The model under review builds one solid part; all positions refer to its coordinate system, in mm. A direction names the side the tool comes from. Coordinates: 2 decimals unless noted, no trailing zeros. Write each loop counter-clockwise with the first axis right and the second up, starting at its lowest first coordinate (ties: lowest second). Pieces come first, ordered by that corner, then holes. Notation, with made-up numbers: (23.5, 75) - (29.5, 75) arc R30 ccw to (29.5, 112) - close; hole circle Ø1 at (56.25, 57). An arc over 180 degrees is marked (long way). Put each result on its own line as item: value.
Autodesk Inventor part; units mm, degrees
ref_plane "YZ Plane" through (0, 0, 0) normal (1, 0, 0) x (0, 1, 0)
ref_plane "XZ Plane" through (0, 0, 0) normal (0, 1, 0) x (-1, 0, 0)
ref_plane "XY Plane" through (0, 0, 0) normal (0, 0, 1) x (1, 0, 0)
sketch "Sketch2" plane through (0, 0, 0) normal (1, 0, 0) x (0, 1, 0)
  line L0 (26.4, -3) -> (6, -3)
  line L1 (6, -3) -> (6, -23.4)
  line L2 (6, -23.4) -> (26.4, -23.4)
  line L3 (26.4, -23.4) -> (26.4, -3)
  line L4 (30.4, 0) -> (0, 0)
  line L5 (30.4, -26.4) -> (30.4, 0)
  line L6 (0, 0) -> (0, -26.4)
  line L7 (30.4, -26.4) -> (0, -26.4)
  line L8 (6, -11) -> (0, -11)
  line L9 (0, -11) -> (0, -15.4)
  line L10 (0, -15.4) -> (6, -15.4)
  line L11 (6, -15.4) -> (6, -11)
  point P0 (0, -11)
  dimension "d5" = 20.4
  dimension "d6" = 20.4
  dimension "d8" = 6
  dimension "d22" = 4
  dimension "d23" = 3
  dimension "d24" = 3
  dimension "d27" = 8
  dimension "d28" = 8
extrude "Extrusion1" add sketch "Sketch2" along normal blind 54.8 contours L0 L1 L8 L6 L4 L5 L7 L10 L2 L3
sketch "Sketch13" plane through (0, 30.4, 0) normal (0, 1, 0) x (1, 0, 0)
  line L0 (0, 0) -> (54.8, 0)
  line L1 (0, 26.4) -> (54.8, 26.4)
  line L2 (54.8, 0) -> (50.8, 0)
  line L3 (50.8, 0) -> (50.8, 26.4)
  line L4 (50.8, 26.4) -> (54.8, 26.4)
  line L5 (54.8, 26.4) -> (54.8, 0)
  line L6 (4, 0) -> (0, 0)
  line L7 (0, 0) -> (0, 26.4)
  line L8 (0, 26.4) -> (4, 26.4)
  line L9 (4, 26.4) -> (4, 0)
  line L10 (0, 26.4) -> (0, 0)
  point P0 (0, 0)
  point P1 (69.8, 0)
  point P2 (69.8, 26.4)
  point P3 (4, 0)
  point P4 (54.8, 26.4)
  point P5 (50.8, 0)
  dimension "d75" = 4
  dimension "d76" = 4
  dimension "d77" = 46.8
extrude "Extrusion11" add sketch "Sketch13" along normal blind 27 contours L7 L1 L9 L0 | L3 L1 L5 L0
sketch "Sketch14" plane through (54.8, 30.4, 0) normal (1, 0, 0) x (0, 0, -1)
  circle A0 centre (5.2, 11) radius 1.3
  circle A1 centre (5.2, 23) radius 1.3
  line L0 (0, -30.4) -> (0, 27)
  circle A2 centre (21.2, 23) radius 1.3
  circle A3 centre (21.2, 11) radius 1.3
  line L1 (26.4, -30.4) -> (26.4, 27)
  line L2 (0, 0) -> (26.4, 0)
  point P0 (26.4, -4)
  dimension "d80" = 2.6
  dimension "d82" = 2.6
  dimension "d86" = 2.6
  dimension "d87" = 2.6
  dimension "d95" = 16
  dimension "d96" = 16
  dimension "d97" = 5.2
  dimension "d98" = 5.2
  dimension "d99" = 5.2
  dimension "d100" = 5.2
  dimension "d101" = 11
  dimension "d102" = 23
extrude "Extrusion12" cut sketch "Sketch14" against normal blind 100
ref_plane "Work Plane1" through (0, 0, -13.2) normal (0, 0, 1) x (1, 0, 0)
sketch "Sketch15" plane through (54.8, 0, 0) normal (1, 0, 0) x (0, 0, -1)
  line L0 (3, 26.4) -> (23.4, 26.4)
  line L1 (26.4, 30.4) -> (0, 30.4)
  line L2 (0, 30.4) -> (26.4, 30.4)
  line L3 (-2.8, 30.4) -> (29.2, 30.4)
  line L4 (29.2, 30.4) -> (29.2, 26.4)
  line L5 (29.2, 26.4) -> (-2.8, 26.4)
  line L6 (-2.8, 26.4) -> (-2.8, 30.4)
  line L7 (13.2, -11.48) -> (13.2, 68.88)
  line L8 (3, 26.4) -> (23.4, 26.4)
  point P0 (0, 0)
  point P1 (13.2, 30.4)
  point P2 (0, 30.4)
  dimension "d103" = 32
extrude "Extrusion13" add sketch "Sketch15" along normal blind 20 and the other way blind 75
sketch "Sketch16" plane through (-20.2, 30.4, 2.8) normal (0, 1, 0) x (1, 0, 0)
  line L0 (0, 32) -> (0, 0)
  line L1 (95, 0) -> (95, 32)
  line L2 (0, 0) -> (95, 0)
  line L3 (95, 0) -> (95, 2.8)
  line L4 (95, 2.8) -> (0, 2.8)
  line L5 (0, 2.8) -> (0, 0)
  line L6 (24.2, 29.2) -> (20.2, 29.2)
  line L7 (20.2, 29.2) -> (20.2, 2.8)
  line L8 (20.2, 2.8) -> (24.2, 2.8)
  line L9 (24.2, 2.8) -> (24.2, 29.2)
  line L10 (75, 29.2) -> (71, 29.2)
  line L11 (71, 29.2) -> (71, 2.8)
  line L12 (71, 2.8) -> (75, 2.8)
  line L13 (75, 2.8) -> (75, 29.2)
  line L14 (0, 0) -> (95, 0)
  line L15 (24.2, 2.8) -> (71, 2.8)
  line L16 (71, 2.8) -> (71, 0)
  line L17 (71, 0) -> (24.2, 0)
  line L18 (24.2, 0) -> (24.2, 2.8)
  point P0 (20.2, 2.8)
  point P1 (71, 2.8)
extrude "Extrusion14" add sketch "Sketch16" along normal blind 27 contours L4 L18 L2 L0 | L16 L4 L1 L2
fillet "Fillet5" radius 3 4 edges at (54.8, 30.4, -13.2) (64.8, 30.4, 0) (0, 30.4, -13.2) (-10.1, 30.4, 0)
sketch "Sketch17" plane through (54.8, 0, 0) normal (1, 0, 0) x (0, 0, -1)
  line L0 (-14.3714, 26.4) -> (47.2508, 26.4)
  line L1 (47.2508, 26.4) -> (47.2508, -4.9204)
  line L2 (47.2508, -4.9204) -> (-14.3714, -4.9204)
  line L3 (-14.3714, -4.9204) -> (-14.3714, 26.4)
  line L4 (-2.8, 26.4) -> (29.2, 26.4)
  point P0 (0, 0)
extrude "Extrusion15" cut sketch "Sketch17" against normal blind 100
equation "\"d98\" = d97"
properties part number "Motor_test_mount"
1. Consider section A-A on z = -21.2. Give the number of separate pieces and of enclosed holes in the cut face, plus the area to 3 significant figures.
Determined:
separate pieces: 5
enclosed holes: 0
area: 558 mm^2
2. To check wall thickness, follow probe 1 along Y at (x, z) = (51, -5); probe 2 along X at (y, z) = (41, -10.5); probe 3 along X at (y, z) = (32, 1). State the ranges of each line that lie inside material, in increasing order.
Determined:
probe 1: y = 26.4 to 40.12, 42.68 to 52.12, 54.68 to 57.4
probe 2: x = 0 to 4, 50.8 to 54.8
probe 3: x = -20.2 to 4, 50.8 to 74.8
3. Machinability: for faces 1 (the cylindrical face through (-0.9, 31.26, -13.02)), 2 (the flat face through (54.8, 45, -13)), 3 (the flat face through (4, 44, -12)), which of the approach directions +Z, -Z, +X, -X, +Y, -Y give a long, thin tool a straight path to every point of the face, cutting with its end or side? Answer none if there is none.
Determined:
face 1: -Z, -X, +Y
face 2: -Z, +X, +Y
face 3: +Z, -Z, +Y
4. For pin 1 Ø2 at (y, z) = (53.4, -21.2) entering from -X; pin 2 Ø8 at (x, y) = (-1, 53.5) entering from -Z; pin 3 Ø4 at (y, z) = (53.4, -5.2) entering from -X; pin 4 Ø16 at (x, z) = (41.5, -11.5) entering from +Y, all flat-tipped, find the tip position at first contact; note any pin that passes through.
Determined:
pin 1: passes through
pin 2: stops at z = -26.4
pin 3: stops at x = 0
pin 4: stops at y = 30.4
5. Consider section B-B on y = 39. State the section outline as (x, z) points.
Determined:
outline: (-20.2, 0) - (0, 0) - (0, -26.4) - (4, -26.4) - (4, 2.8) - (-20.2, 2.8) - close; (50.8, -26.4) - (54.8, -26.4) - (54.8, 0) - (74.8, 0) - (74.8, 2.8) - (50.8, 2.8) - close
6. Consider section D-D on x = 62.5. State the section outline as (y, z) points, plus the area to 3 significant figures.
Determined:
outline: (26.4, -29.2) - (30.4, -29.2) - (30.4, -3) arc R3 cw to (33.4, 0) - (57.4, 0) - (57.4, 2.8) - (26.4, 2.8) - close
area: 206 mm^2
7. Consider section C-C on x = 3. State the section outline as (y, z) points.
Determined:
outline: (26.4, -29.2) - (30.4, -29.2) - (30.4, -26.4) - (57.4, -26.4) - (57.4, 2.8) - (26.4, 2.8) - close; hole circle Ø2.6 at (41.4, -21.2); hole circle Ø2.6 at (41.4, -5.2); hole circle Ø2.6 at (53.4, -21.2); hole circle Ø2.6 at (53.4, -5.2)
8. The part is to be moulded in two halves that separate along Z. For faces 4 (the flat face through (27, 28, -29.2)), 5 (the cylindrical face through (2.028, 52.247, -21.8)), 6 (the flat face through (50.8, 44, -12)), say which applies: +Z half, -Z half, draft (parallel to the pull), parting line (faces both ways), or undercut.
Determined:
face 4: -Z half
face 5: undercut
face 6: draft
